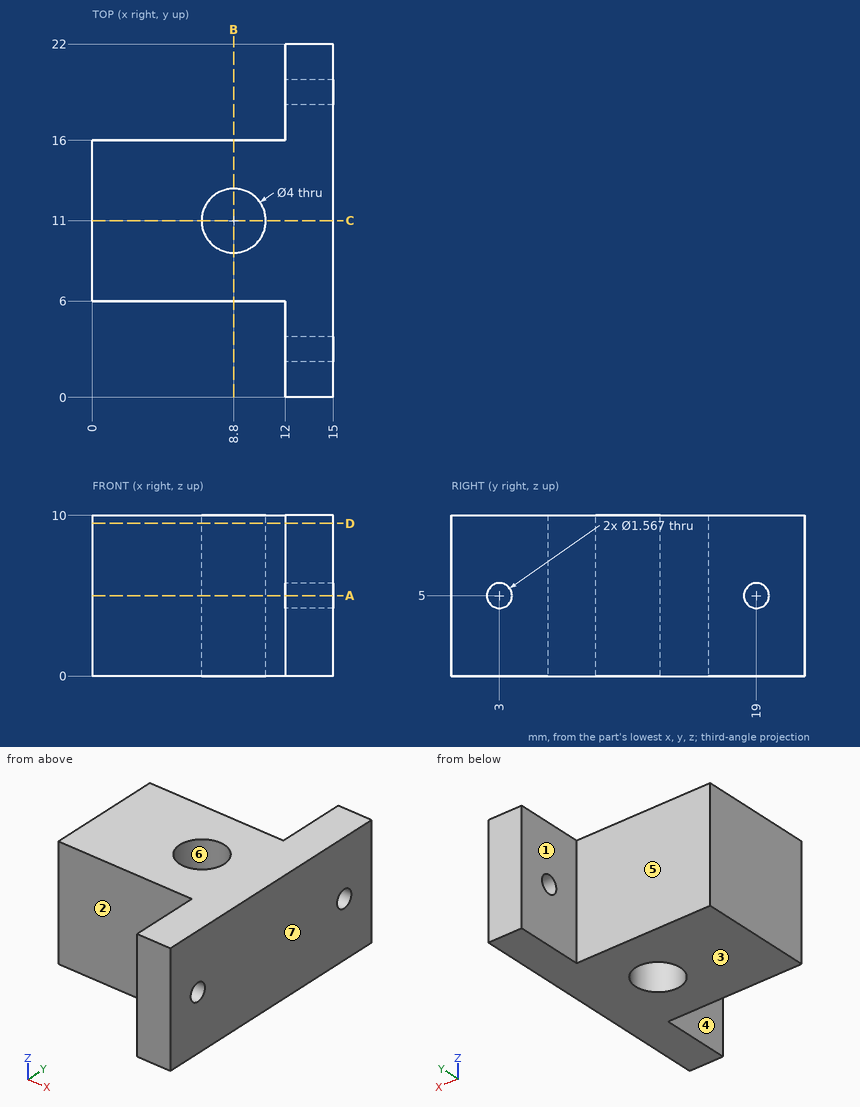
Geometry check sheet. Reference: drawing and pictorial views, mm from the part's lowest x, y, z. A direction names the side the tool comes from. Give positions to 0.01 mm unless a question says otherwise; leave off trailing zeros. Order: outer loops, then holes, each group sorted by start corner. A loop starts at its lowest first (then second) coordinate and runs counter-clockwise, first axis right, second up. Notation, with made-up numbers: (51.25, -40) - (71.25, -40) arc R8 ccw to (71.25, -26) - close; hole circle Ø6 at (63.25, 89). An arc over 180 degrees is marked (long way). Use one line per item in the form item = value.
1) Access from +Z, -Z, +X, -X, +Y, -Y to the whole of each face (thin tool, end or side, straight path). Record for the marked faces 1, 2 and 3.
Working result:
face_1 = +Z, -Z, -X, +Y
face_2 = +Z, -Z, -X, -Y
face_3 = -Z, +X, -X, +Y, -Y
2) Draft check along X on the marked faces 4, 5, 6 and 7. Enter one of: released by +X, released by -X, zero draft, split by the parting line, or undercut.
Working result:
face_4 = released by -X
face_5 = zero draft
face_6 = undercut
face_7 = released by +X
3) Sectioned sample at C-C (y = 11). Record the boundary of the cut face in (x, z).
Working result:
outline = (0, 0) - (6.8, 0) - (6.8, 10) - (0, 10) - close; (10.8, 0) - (15, 0) - (15, 10) - (10.8, 10) - close
4) Sectioned sample at A-A (z = 5). Record the boundary of the cut face in (x, y), and give its area (3 significant figures).
Working result:
outline = (0, 6) - (12, 6) - (12, 3.78) - (15, 3.78) - (15, 18.22) - (12, 18.22) - (12, 16) - (0, 16) - close; (12, 0) - (15, 0) - (15, 2.22) - (12, 2.22) - close; (12, 19.78) - (15, 19.78) - (15, 22) - (12, 22) - close; hole circle Ø4 at (8.8, 11)
area = 164 mm^2
5) Sectioned sample at B-B (x = 8.8). Record the boundary of the cut face in (y, z).
Working result:
outline = (6, 0) - (9, 0) - (9, 10) - (6, 10) - close; (13, 0) - (16, 0) - (16, 10) - (13, 10) - close
6) Material ranges on probe 1 along Y at (x, z) = (14, 5); probe 2 along X at (y, z) = (19.5, 1); probe 3 along Y at (x, z) = (3, 8), recorded low to high. Write a range as from..to.
Working result:
probe_1 = 0..2.22, 3.78..18.22, 19.78..22
probe_2 = 12..15
probe_3 = 6..16
7) Depth check by flat-ended pin: pin 1 Ø4 at (x, z) = (2.5, 4.5) entering from +Y; pin 2 Ø1.4 at (y, z) = (3, 5) entering from +X; pin 3 Ø3 at (y, z) = (3.5, 7) entering from -X. Enter the tip coordinate at first touch or a pass-through.
Working result:
pin_1 = 16
pin_2 = through
pin_3 = 12
8) Sectioned sample at D-D (z = 9.5). Record the boundary of the cut face in (x, y).
Working result:
outline = (0, 6) - (12, 6) - (12, 0) - (15, 0) - (15, 22) - (12, 22) - (12, 16) - (0, 16) - close; hole circle Ø4 at (8.8, 11)
